from build123d import *

# Parameters (mm, degrees)
SKETCH1_W           = 48.26
SKETCH1_H           = 25.5651
BOSS_EXTRUDE1_DEPTH = 17.78
SHELL1_T            = -2.54
SKETCH2_R           = 3.175
BOSS_EXTRUDE2_DEPTH = 25.4
BOSS_EXTRUDE3_DEPTH = 12.7


with BuildPart() as part:
    # Sketch1 → Boss-Extrude1 (new, symmetric)
    with BuildSketch(Plane.XY):
        with Locations((24.13, -12.78255)):
            Rectangle(SKETCH1_W, SKETCH1_H)
    extrude(amount=BOSS_EXTRUDE1_DEPTH, both=True)

    # Shell1
    shell1_openings = [part.faces().sort_by_distance(p)[0] for p in [
        (24.13, -25.5651, 0),
    ]]
    offset(amount=SHELL1_T, openings=shell1_openings, kind=Kind.INTERSECTION)

    # Sketch2 → Boss-Extrude2 (add)
    with BuildSketch(Plane.XZ.offset(2.54)):
        with Locations(Location((27.94, 0, 0), (0, 0, 90))):
            Circle(SKETCH2_R)
    extrude(amount=BOSS_EXTRUDE2_DEPTH)

    # Sketch3 → Boss-Extrude3 (add, symmetric)
    with BuildSketch(Plane.XY):
        with BuildLine():
            Line((1.27, -25.5651), (2.54, -25.5651))
            Line((2.54, -25.5651), (2.54, -30.6451))
            Line((2.54, -30.6451), (1.27, -30.6451))
            ThreePointArc((1.27, -30.6451), (0, -29.3751), (1.27, -28.1051))
            Line((1.27, -28.1051), (1.27, -25.5651))
        make_face()
        with BuildLine():
            Line((45.72, -25.5651), (45.72, -30.6451))
            Line((45.72, -30.6451), (46.99, -30.6451))
            ThreePointArc((46.99, -30.6451), (48.26, -29.3751), (46.99, -28.1051))
            Line((46.99, -28.1051), (46.99, -25.5651))
            Line((46.99, -25.5651), (45.72, -25.5651))
        make_face()
    extrude(amount=BOSS_EXTRUDE3_DEPTH, both=True)


solid = part.part
Model file for the job. Use its own axes, mm. A direction names the side the tool comes from. Give positions to 0.01 mm unless a question says otherwise; leave off trailing zeros. Order: outer loops, then holes, each group sorted by start corner. A loop starts at its lowest first (then second) coordinate and runs counter-clockwise, first axis right, second up. Notation, with made-up numbers: (78.25, 69) - (90.25, 69) arc R21 ccw to (90.25, 107) - close; hole circle Ø4 at (-34.5, -2.75). An arc over 180 degrees is marked (long way). Return JSON: item names as keys, results as strings.
1) Pull direction X, two halves, no side cores. Call faces 1 (the flat face through (45.72, -17, 0)), 2 (the flat face through (2, -30.645, 0)), 3 (the flat face through (1.27, -27, 0)): pulls with the +X half, pulls with the -X half, needs draft (parallel to the pull), parting line crosses it, or undercut.
Geometry says:
{"face 1": "undercut", "face 2": "needs draft", "face 3": "pulls with the -X half"}
2) Cut at B-B, the plane z = -5. Give the cut face in (x, y).
Geometry says:
{"outline": "(0, -25.57) - (1.27, -25.57) - (1.27, -28.11) arc R1.27 ccw to (1.27, -30.65) - (2.54, -30.65) - (2.54, -2.54) - (45.72, -2.54) - (45.72, -30.65) - (46.99, -30.65) arc R1.27 ccw to (46.99, -28.11) - (46.99, -25.57) - (48.26, -25.57) - (48.26, 0) - (0, 0) - close"}
3) Cut at D-D, the plane z = -14. Give the cut face in (x, y), plus the area to 3 significant figures.
Geometry says:
{"outline": "(0, -25.57) - (2.54, -25.57) - (2.54, -2.54) - (45.72, -2.54) - (45.72, -25.57) - (48.26, -25.57) - (48.26, 0) - (0, 0) - close", "area": "240 mm²"}
4) Cut at A-A, the plane y = -10.5. Give the cut face in (x, z) (3 decimals), plus the area to 3 significant figures.
Geometry says:
{"outline": "(0, -17.78) - (48.26, -17.78) - (48.26, 17.78) - (0, 17.78) - close; circle Ø6.35 at (27.94, 0); hole (2.54, -15.24) - (45.72, -15.24) - (45.72, 15.24) - (2.54, 15.24) - close", "area": "432 mm²"}
5) Flat gauge pins, fed straight in: P1, Ø0.8, axis at x = 47, y = -27.5, coming from the +Z side; P2, Ø1.9, axis at x = 27.5, z = 0, coming from the -Y side; P3, Ø1.3, axis at y = -26.5, z = 4.5, coming from the +X side. Where does each tip first touch, or does it go through?
Geometry says:
{"P1": "z = 12.7", "P2": "y = -27.94", "P3": "x = 46.99"}
6) Cut at C-C, the plane x = 27.94. Give the cut face in (y, z) (3 decimals), plus the area to 3 significant figures.
Geometry says:
{"outline": "(-27.94, -3.175) - (-2.54, -3.175) - (-2.54, -15.24) - (-25.565, -15.24) - (-25.565, -17.78) - (0, -17.78) - (0, 17.78) - (-25.565, 17.78) - (-25.565, 15.24) - (-2.54, 15.24) - (-2.54, 3.175) - (-27.94, 3.175) - close", "area": "369 mm²"}
7) Probe line 1 (X direction, y = -22.5, z = 0) (3 decimals); line 2 (X direction, y = -12.5, z = 13); line 3 (Z direction, x = 33.5, y = -24). List the from-to ranges inside material, lowest first. Write a range as from..to.
Geometry says:
{"line 1": "0..2.54, 24.765..31.115, 45.72..48.26", "line 2": "0..2.54, 45.72..48.26", "line 3": "-17.78..-15.24, 15.24..17.78"}
8) 3-axis set-ups, long thin cutter, end or side, ignore diameter. For faces 4 (the flat face through (2, -29, 12.7)), 5 (the flat face through (46.99, -27, 0)), 6 (the flat face through (24, -14, 15.24)), 7 (the flat face through (2, -29, -12.7)), 8 (the flat face through (28, -27.94, 0)): which of +Z, -Z, +X, -X, +Y, -Y reach the whole face in a straight line?
Geometry says:
{"face 4": "+Z, +X, -X, -Y", "face 5": "+Z, -Z, +X", "face 6": "-Y", "face 7": "-Z, +X, -X, -Y", "face 8": "+Z, -Z, -Y"}
